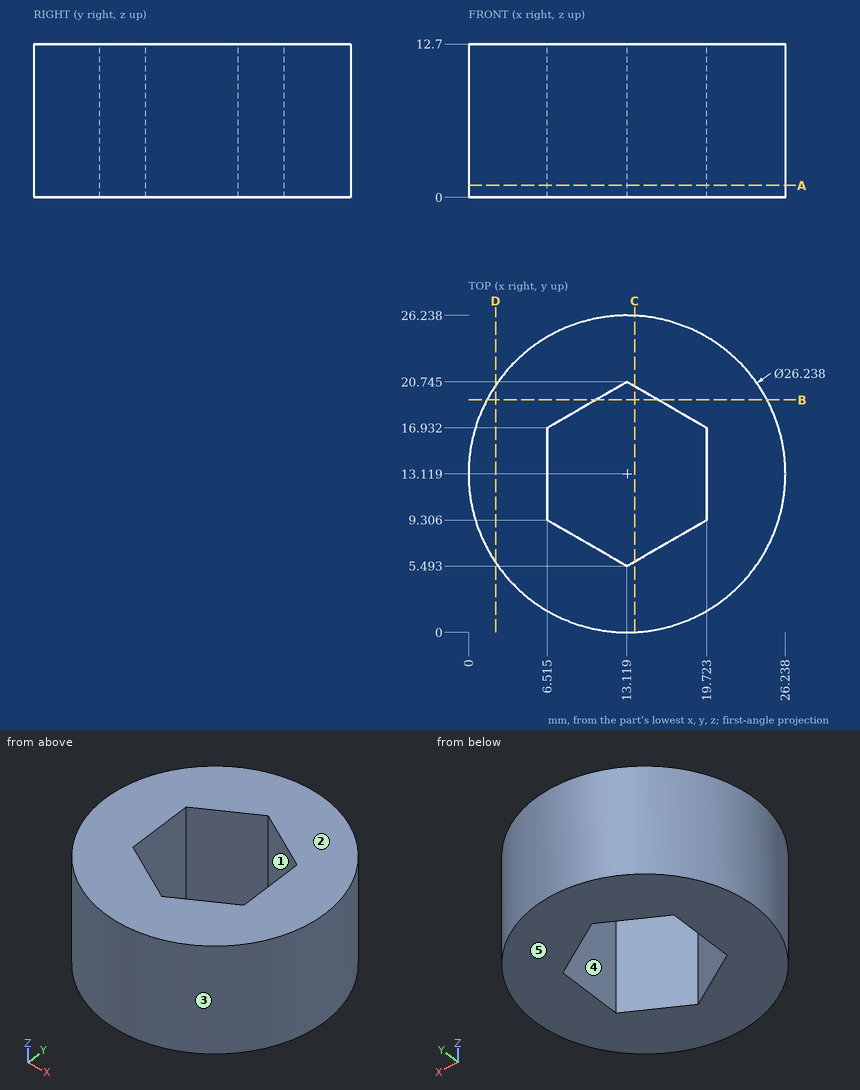
Answer from the drawing. Dimensions are ordinates in mm from the lowest x, y and z of the part. A direction names the side the tool comes from. Coordinates: 2 decimals unless noted, no trailing zeros. Loops run counter-clockwise (first coordinate to the right, second up) from the corner with the lowest first, then second, coordinate; pieces in that order, holes last. Notation, with made-up numbers: (88.5, -2) -> (125.5, -2) arc R32 cw to (125.5, 33) -> close; hole circle Ø10 at (-26.5, 16.5). An arc over 180 degrees is marked (long way). Return JSON: item names as keys, results as strings.
Item 1: Find section A-A (z = 1). Determine the outline of the cut face in (x, y) (1 decimal), plus the area to 3 significant figures.
Answers:
{"outline": "circle Ø26.2 at (13.1, 13.1); hole (6.5, 9.3) -> (13.1, 5.5) -> (19.7, 9.3) -> (19.7, 16.9) -> (13.1, 20.7) -> (6.5, 16.9) -> close", "area": "390 mm2"}
Item 2: For the marked faces 1 and 2, determine the directions among +Z, -Z, +X, -X, +Y, -Y from which every point of the face is accessible in a straight line to the end or side of a thin tool.
Answers:
{"face 1": "+Z, -Z", "face 2": "+Z, +X, -X, +Y, -Y"}
Item 3: For a pull along X with two mould halves and no side action, classify the marked faces 3, 4 and 5 as +X half, -X half, draft (parallel to the pull), parting line (faces both ways), or undercut.
Answers:
{"face 3": "parting line", "face 4": "undercut", "face 5": "draft"}
Item 4: Find section B-B (y = 19.25). Determine the outline of the cut face in (x, z).
Answers:
{"outline": "(1.52, 0) -> (10.53, 0) -> (10.53, 12.7) -> (1.52, 12.7) -> close; (15.71, 0) -> (24.72, 0) -> (24.72, 12.7) -> (15.71, 12.7) -> close"}
Item 5: Find section D-D (x = 2.25). Determine the outline of the cut face in (y, z) (1 decimal), plus the area to 3 significant figures.
Answers:
{"outline": "(5.8, 0) -> (20.5, 0) -> (20.5, 12.7) -> (5.8, 12.7) -> close", "area": "187 mm2"}
Item 6: Flat-ended cylindrical pins translate along their axes: P1, Ø6, axis at y = 6, z = 11, coming from the +X side (1 decimal); P2, Ø4, axis at y = 18, z = 2, coming from the -X side; P3, Ø3, axis at x = 23, z = 3, coming from the +Y side. Find the tip coordinate at first contact, or state that the pin passes through.
Answers:
{"P1": "stops at x = 25.6", "P2": "stops at x = 0.32", "P3": "stops at y = 23.21"}
Item 7: Find the intervals of material crossed by probe 1 along Y at (x, z) = (13.5, 1.5) (1 decimal); probe 2 along X at (y, z) = (9.75, 10) (1 decimal); probe 3 along Y at (x, z) = (11.75, 5.25) (1 decimal), in increasing order.
Answers:
{"probe 1": "y = 0 to 5.7, 20.5 to 26.2", "probe 2": "x = 0.4 to 6.5, 19.7 to 25.8", "probe 3": "y = 0.1 to 6.3, 20 to 26.2"}
Item 8: Find section C-C (x = 13.75). Determine the outline of the cut face in (y, z) (1 decimal).
Answers:
{"outline": "(0, 0) -> (5.9, 0) -> (5.9, 12.7) -> (0, 12.7) -> close; (20.4, 0) -> (26.2, 0) -> (26.2, 12.7) -> (20.4, 12.7) -> close"}
